Part model, mm, in its own coordinate system. Face numbers are marked on the shaded views. A direction names the side the tool comes from. Give positions to 0.01 mm unless a question says otherwise; leave off trailing zeros. Order: outer loops, then holes, each group sorted by start corner. A loop starts at its lowest first (then second) coordinate and runs counter-clockwise, first axis right, second up. Notation, with made-up numbers: M 16.5,57.5 L 41.5,57.5 A3 cw 41.5,61.5 Z; hole C 49,-11.5 d10. An arc over 180 degrees is marked long. Write each question's results on one line, items separated by ' | '. Start each with the question number.
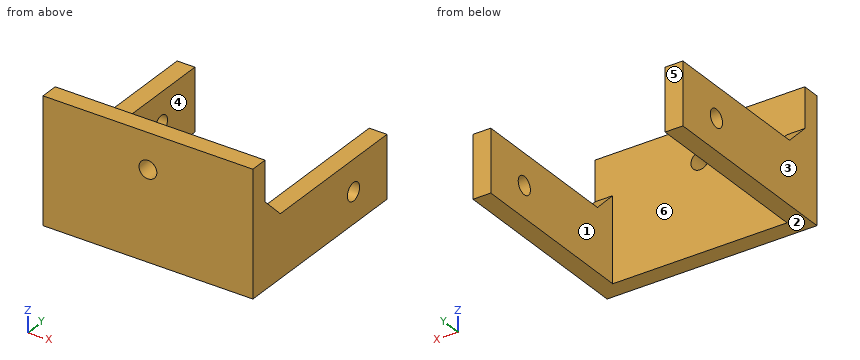
from build123d import *

# Parameters (mm, degrees)
SKETCH1_W           = 23.6
SKETCH1_H           = 14
BOSS_EXTRUDE1_DEPTH = 2
BOSS_EXTRUDE2_DEPTH = 2
BOSS_EXTRUDE3_DEPTH = 2
SKETCH4_R           = 1
CUT_EXTRUDE1_DEPTH  = 2
SKETCH5_R           = 1
CUT_EXTRUDE2_DEPTH  = 34.01454225


with BuildPart() as part:
    # Sketch1 → Boss-Extrude1 (new body)
    with BuildSketch(Plane(origin=(0, 0, 0), x_dir=(1, 0, 0), z_dir=(0, 1, 0))):
        Rectangle(SKETCH1_W, SKETCH1_H)
    extrude(amount=BOSS_EXTRUDE1_DEPTH)

    # Sketch2 → Boss-Extrude2 (add)
    with BuildSketch(Plane(origin=(11.8, 0, 0), x_dir=(0, 0, -1), z_dir=(1, 0, 0))):
        Polygon((7, 2), (0, 2), (-2.5, 2), (0, 4.5), (0, 22), (7, 22), align=None)
    extrude(amount=-BOSS_EXTRUDE2_DEPTH)

    # Sketch3 → Boss-Extrude3 (add)
    with BuildSketch(Plane.ZY.offset(11.8)):
        Polygon((-7, 22), (-7, 2), (2.5, 2), (0, 4.5), (0, 22), align=None)
    extrude(amount=-BOSS_EXTRUDE3_DEPTH)

    # Sketch4 → Cut-Extrude1 (cut)
    with BuildSketch(Plane.XZ):
        with Locations(Location((0, 3, 0), (0, 0, 270))):
            Circle(SKETCH4_R)
    extrude(amount=-CUT_EXTRUDE1_DEPTH, mode=Mode.SUBTRACT)

    # Sketch5 → Cut-Extrude2 (cut, through all)
    with BuildSketch(Plane(origin=(11.8, 0, 0), x_dir=(0, 0, -1), z_dir=(1, 0, 0))):
        with Locations((3.5, 16.5)):
            Circle(SKETCH5_R)
    extrude(amount=-CUT_EXTRUDE2_DEPTH, mode=Mode.SUBTRACT)


solid = part.part
(1) Drop flat-ended pins along their axis: P1, Ø10, axis at x = 3.5, y = 10.5, coming from the -Z side; P2, Ø2, axis at x = -10.5, y = 9.5, coming from the +Z side; P3, Ø7, axis at x = 4, z = 0, coming from the +Y side. Give the stop position or say it passes through.
(2) Pull direction X, two halves, no side cores. Call the marked faces 3, 4, 5 and 6: +X half, -X half, draft (parallel to the pull), parting line (faces both ways), or undercut.
(3) Saw through at A-A on y = 16.5. Give the cut face in (x, z), plus the area to 3 significant figures.
(4) Probe L1, parallel to Y at x = -10.25, z = -3.5; L2, parallel to X at y = 20.5, z = -3.5; L3, parallel to X at y = 1.65, z = 3. List the from-to ranges inside material, lowest first.
(5) Saw through at B-B on z = 3. Give the cut face in (x, y), plus the area to 3 significant figures.
(6) Saw through at C-C on x = 0. Give the cut face in (y, z), plus the area to 3 significant figures.
(7) Saw through at D-D on z = -3.5. Give the cut face in (x, y).
(8) Tool access for the marked faces 1 and 2: list every direction of +Z, -Z, +X, -X, +Y, -Y with a clear straight run to the whole face (end or side of a thin tool).
Taken from the geometry:
1) P1: passes through | P2: stops at z = 0 | P3: stops at y = 2
2) face 3: -X half | face 4: undercut | face 5: draft | face 6: undercut
3) outline: M -11.8,-7 L -9.8,-7 L -9.8,-4.5 L -11.8,-4.5 Z; M -11.8,-2.5 L -9.8,-2.5 L -9.8,0 L -11.8,0 Z; M 9.8,-7 L 11.8,-7 L 11.8,-4.5 L 9.8,-4.5 Z; M 9.8,-2.5 L 11.8,-2.5 L 11.8,0 L 9.8,0 Z | area: 20.0 mm²
4) L1: y = 0 to 15.5, 17.5 to 22 | L2: x = -11.8 to -9.8, 9.8 to 11.8 | L3: x = -11.8 to -1, 1 to 11.8
5) outline: M -11.8,0 L -1,0 L -1,2 L -11.8,2 Z; M 1,0 L 11.8,0 L 11.8,2 L 1,2 Z | area: 43.2 mm²
6) outline: M 0,-7 L 2,-7 L 2,2 L 0,2 Z; M 0,4 L 2,4 L 2,7 L 0,7 Z | area: 24.0 mm²
7) outline: M -11.8,0 L 11.8,0 L 11.8,15.5 L 9.8,15.5 L 9.8,2 L -9.8,2 L -9.8,15.5 L -11.8,15.5 Z; M -11.8,17.5 L -9.8,17.5 L -9.8,22 L -11.8,22 Z; M 9.8,17.5 L 11.8,17.5 L 11.8,22 L 9.8,22 Z
8) face 1: +Z, -Z, +Y | face 2: -Z, +X, -X, +Y, -Y
